Input: part model. Units: mm. Frame: model coordinates. Give positions to 0.01 mm unless a question says otherwise; leave off trailing zeros. Loops run counter-clockwise (first coordinate to the right, second up) from the corner with the lowest first, then second, coordinate; pieces in that order, holes last. Notation, with made-up numbers: M 77,21 L 105,21 A21 ccw 105,53 Z; hole C 51,41.5 d1. An arc over 180 degrees is marked long. Answer as a JSON object with one key per item and string values. Group by question number.
1) Ray query, L1, parallel to Z at x = 0, y = 3.15; L2, parallel to Z at x = 2.75, y = 0.55; L3, parallel to X at y = 1.8, z = 2.75. Return the intervals inside material, ascending.
2) First-contact query: P1, Ø5.5, axis at x = 0, z = 0, coming from the -Y side. Flat tip, straight axial feed; report the tip coordinate or a pass-through.
3) Draft query along Z for faces 1 (the cylindrical face through (3, 2, 0)), 2 (the conical face through (2.605, 4.812, 4.487)), 3 (the conical face through (2.583, 4.812, -4.499)). Return one class per face: +Z half, -Z half, draft (parallel to the pull), parting line (faces both ways), or undercut.
4) Section query A-A on y = 1.05. Return loops of the section in (x, z).
Autodesk Inventor part; units mm, degrees
ref_plane "YZ Plane" through (0, 0, 0) normal (1, 0, 0) x (0, 1, 0)
ref_plane "XZ Plane" through (0, 0, 0) normal (0, 1, 0) x (-1, 0, 0)
ref_plane "XY Plane" through (0, 0, 0) normal (0, 0, 1) x (1, 0, 0)
sketch "Esboço1" plane through (0, 0, 0) normal (0, 1, 0) x (-1, 0, 0)
  circle A0 centre (0, 0) radius 3
  line L0 (-2.8868, -5) -> (-5.7735, 0)
  line L1 (-5.7735, 0) -> (-2.8868, 5)
  line L2 (-2.8868, 5) -> (2.8868, 5)
  line L3 (2.8868, 5) -> (5.7735, 0)
  line L4 (5.7735, 0) -> (2.8868, -5)
  line L5 (2.8868, -5) -> (-2.8868, -5)
  dimension "d0" = 6
extrude "Extrusão1" add sketch "Esboço1" along normal blind 5
thread "Rosca1"
sketch "Esboço2" plane through (0, 0, 0) normal (1, 0, 0) x (0, 1, 0)
  point P0 (0, 0)
chamfer "Chanfro1" distance 0.5 angle 45 2 edges at (3, 0, 0) (3, 5, 0)
sketch "Esboço5" plane through (0, 0, 0) normal (0, -1, 0) x (1, 0, 0)
  circle A0 centre (0, 0) radius 5
extrude "Extrusão2" cut sketch "Esboço5" against normal through all draft 45 keep common part
sketch "Esboço6" plane through (0, 5, 0) normal (0, 1, 0) x (1, 0, 0)
  circle A0 centre (0, 0) radius 5
extrude "Extrusão3" cut sketch "Esboço6" against normal through all draft 45 keep common part
properties part number "porca m6" material "Aço inoxidável"
Output:
{
 "1": {"L1": "z = -5 to -3, 3 to 5", "L2": "z = -4.82 to -1.2, 1.2 to 4.82", "L3": "x = -4.19 to -1.2, 1.2 to 4.19"},
 "2": {"P1": "passes through"},
 "3": {"face 1": "undercut", "face 2": "+Z half", "face 3": "-Z half"},
 "4": {"outline": "M -5.77,0 L -2.89,-5 L 2.89,-5 L 5.77,0 L 2.89,5 L -2.89,5 Z; hole C 0,0 d6"}
}
